Here's how the part is built. I have some questions about the finished solid (model axes, mm). Round coordinates to 2 decimals unless told otherwise and drop trailing zeros. Order: outer loops, then holes, each group sorted by start corner. A loop starts at its lowest first (then second) coordinate and runs counter-clockwise, first axis right, second up. Notation, with made-up numbers: (61, -1.75) -> (87, -1.75) arc R30 ccw to (87, 28.25) -> close; hole circle Ø11 at (23, 66). An arc over 180 degrees is marked (long way). Answer in a Markdown table with one row per item.
```python
from build123d import *

# Parameters (mm, degrees)
SKETCH1_R           = 2.54
BOSS_EXTRUDE1_DEPTH = 2.54


with BuildPart() as part:
    # Sketch1 → Boss-Extrude1 (new body)
    # profile 1 of 3: a face of its own
    with BuildSketch(Plane(origin=(0, 0, 0), x_dir=(0, 0, -1), z_dir=(1, 0, 0))):
        with BuildLine():
            ThreePointArc((-263.315482234, 15.875), (-252.090162082, 11.225320151), (-247.440482234, 0))
            ThreePointArc((-247.440482234, 0), (-250.845779802, -9.824568503), (-259.600752631, -15.434260882))
            ThreePointArc((-259.600752631, -15.434260882), (3.384517766, 0.002547972), (266.369788164, -15.434260882))
            ThreePointArc((266.369788164, -15.434260882), (254.320087607, 1.870392137), (270.084517766, 15.875))
            ThreePointArc((270.084517766, 15.875), (3.384517766, 42.576584001), (-263.315482234, 15.875))
        make_face()
    # profile 2 of 3: a face of its own
    with BuildSketch(Plane(origin=(0, 0, 0), x_dir=(0, 0, -1), z_dir=(1, 0, 0))):
        with BuildLine():
            ThreePointArc((-259.600752631, -15.434260882), (-250.845779802, -9.824568503), (-247.440482234, 0))
            ThreePointArc((-247.440482234, 0), (-252.090162082, 11.225320151), (-263.315482234, 15.875))
            ThreePointArc((-263.315482234, 15.875), (-279.190482234, 0), (-263.315482234, -15.875))
            ThreePointArc((-263.315482234, -15.875), (-261.458209114, -15.653857706), (-259.600752631, -15.434260882))
        make_face()
        with Locations((-263.315482234, 0)):
            Circle(SKETCH1_R, mode=Mode.SUBTRACT)
    # profile 3 of 3: a face of its own
    with BuildSketch(Plane(origin=(0, 0, 0), x_dir=(0, 0, -1), z_dir=(1, 0, 0))):
        with BuildLine():
            ThreePointArc((285.959517766, 0), (281.309837918, 11.225320151), (270.084517766, 15.875))
            ThreePointArc((270.084517766, 15.875), (254.320087607, 1.870392137), (266.369788164, -15.434260882))
            ThreePointArc((266.369788164, -15.434260882), (268.227244647, -15.653857706), (270.084517766, -15.875))
            ThreePointArc((270.084517766, -15.875), (281.309837918, -11.225320151), (285.959517766, 0))
        make_face()
        with Locations((270.084517766, 0)):
            Circle(SKETCH1_R, mode=Mode.SUBTRACT)
    extrude(amount=BOSS_EXTRUDE1_DEPTH)


solid = part.part
```
1. We'd pull the mould along Z, two halves only. Please class faces 1 (the face through (1.252, 0.349, 279.187)), 2 (the face through (1, 0, 0)), 3 (the face through (0, 14, 1)): released by +Z, released by -Z, zero draft, split by the parting line, or undercut.
Numbers:
| item | result |
|---|---|
| face 1 | released by +Z |
| face 2 | undercut |
| face 3 | zero draft |
2. Suppose I cut it at B-B on z = -104. Write out the boundary of the cut face in (x, y), then the cut area to 3 significant figures.
Numbers:
| item | result |
|---|---|
| outline | (0, -2.25) -> (2.54, -2.25) -> (2.54, 38.81) -> (0, 38.81) -> close |
| area | 104 mm2 |
3. Please list where these lines run through material, in increasing order: line 1 along Y through (x, z) = (1.8, -18); line 2 along Y through (x, z) = (2, 193.5); line 3 along Z through (x, y) = (0.3, 13).
Numbers:
| item | result |
|---|---|
| line 1 | y = -0.04 to 42.5 |
| line 2 | y = -8.64 to 28.09 |
| line 3 | z = -279.2 to 272.43 |
4. For pin 1 Ø1.5 at (x, z) = (1.5, 178) entering from -Y, with a flat end and sliding along its axis, tell me the tip position at first contact or that it passes through.
Numbers:
| item | result |
|---|---|
| pin 1 | stops at y = -7.39 |
5. Suppose I cut it at A-A on x = 1.6. Write out the boundary of the cut face in (y, z) (3 decimals).
Numbers:
| item | result |
|---|---|
| outline | (-15.875, -270.085) arc R15.875 ccw to (15.875, -270.085) arc R1345.273 ccw to (15.875, 263.315) arc R15.875 ccw to (-15.875, 263.315) arc R2247.861 cw to (-15.434, 259.601) arc R2247.859 cw to (-15.434, -266.37) arc R2247.861 cw to start; hole circle Ø5.08 at (0, -270.085); hole circle Ø5.08 at (0, 263.315) |
